Work out the finished part from the listing and answer in its coordinate system (mm). A direction names the side the tool comes from. Round coordinates to 2 decimals unless told otherwise and drop trailing zeros. Write each loop counter-clockwise with the first axis right and the second up, starting at its lowest first coordinate (ties: lowest second). Pieces come first, ordered by that corner, then holes.
1. Determine the mould class of faces 1 (the face through (-6.889, -8.376, 1.479)), 2 (the face through (15.021, -7.951, 28.248)), 3 (the face through (-2, -1, 3)), 4 (the face through (-10.907, 15.021, 28.248)) for opening direction Z: pulls with the +Z half, pulls with the -Z half, needs draft (parallel to the pull), parting line crosses it, or undercut.
2. Flat-ended cylindrical pins translate along their axes: pin 1 Ø9 at (y, z) = (4, 17) entering from -X; pin 2 Ø2 at (x, z) = (-5.5, 13) entering from -Y; pin 3 Ø5 at (x, y) = (-9.43, -9.43) entering from -Z. Find the tip coordinate at first contact, or state that the pin passes through.
3. Find section A-A (x = -9). Write down the section's boundary in (y, z), and give its area (3 significant figures).
4. Find section D-D (z = 6). Write down the section's boundary in (x, y).
5. Find section B-B (y = -7.5). Write down the section's boundary in (x, z), and give its area (3 significant figures).
6. Straight lines are drawn through the part: probe 1 along X at (y, z) = (-1, 15); probe 2 along Z at (x, y) = (-3, 5.5). For each, find the intervals that lie inside material, in ascending order.
7. A tool of negligible diameter and unlimited length cuts with its end or side. For faces 5 (the face through (0, 0, 0)), 6 (the face through (13.5, -2, 18)), from which of +Z, -Z, +X, -X, +Y, -Y can it reach the whole face along a straight path? Write none if from no direction.
8. Find section C-C (x = -3). Write down the section's boundary in (y, z).
```python
from build123d import *

# Parameters (mm, degrees)
F0_W     = 33
F0_H     = 33
F1_DEPTH = 3
F2_W     = 30
F2_H     = 3
F2_W_2   = 3
F2_H_2   = 30
F3_DEPTH = 30
F6_R     = 2.75
F7_DEPTH = 3
F4_R     = 2.75
F8_DEPTH = 3
F5_R     = 2.75
F9_DEPTH = 3


with BuildPart() as f1:
    # F0 (on Top) → F1 (new body)
    with BuildSketch(Plane.XY):
        Rectangle(F0_W, F0_H)
    extrude(amount=F1_DEPTH)

    # F2 (on face) → F3 (join)
    with BuildSketch(Plane.XY.offset(3)):
        with Locations((-1.5, 15)):
            Rectangle(F2_W, F2_H)
        with Locations((15, 15)):
            Rectangle(F2_W_2, F2_H)
        with Locations((15, -1.5)):
            Rectangle(F2_W_2, F2_H_2)
    extrude(amount=F3_DEPTH)

    # F6 (on face) → F7 (cut)
    with BuildSketch(Plane(origin=(0, 16.5, 0), x_dir=(-1, 0, 0), z_dir=(0, 1, 0))):
        with Locations((9.428932, 25.928932)):
            Circle(F6_R)
    extrude(amount=-F7_DEPTH, mode=Mode.SUBTRACT)

    # F4 (on face) → F8 (cut)
    with BuildSketch(Plane(origin=(0, 0, 0), x_dir=(1, 0, 0), z_dir=(0, 0, -1))):
        with Locations((-9.428932, 9.428932)):
            Circle(F4_R)
    extrude(amount=-F8_DEPTH, mode=Mode.SUBTRACT)

    # F5 (on face) → F9 (cut)
    with BuildSketch(Plane.YZ.offset(16.5)):
        with Locations((-9.428932, 25.928932)):
            Circle(F5_R)
    extrude(amount=-F9_DEPTH, mode=Mode.SUBTRACT)


solid = f1.part
```
Worked answers:
1. face 1: needs draft
1. face 2: undercut
1. face 3: pulls with the +Z half
1. face 4: undercut
2. pin 1: stops at x = 13.5
2. pin 2: stops at y = 13.5
2. pin 3: passes through
3. outline: (-16.5, 0) - (-12.15, 0) - (-12.15, 3) - (-16.5, 3) - close; (-6.71, 0) - (16.5, 0) - (16.5, 23.21) - (13.5, 23.21) - (13.5, 3) - (-6.71, 3) - close; (13.5, 28.65) - (16.5, 28.65) - (16.5, 33) - (13.5, 33) - close
3. area: 156 mm2
4. outline: (-16.5, 13.5) - (13.5, 13.5) - (13.5, -16.5) - (16.5, -16.5) - (16.5, 16.5) - (-16.5, 16.5) - close
5. outline: (-16.5, 0) - (-11.39, 0) - (-11.39, 3) - (-16.5, 3) - close; (-7.47, 0) - (16.5, 0) - (16.5, 23.97) - (13.5, 23.97) - (13.5, 3) - (-7.47, 3) - close; (13.5, 27.89) - (16.5, 27.89) - (16.5, 33) - (13.5, 33) - close
5. area: 165 mm2
6. probe 1: x = 13.5 to 16.5
6. probe 2: z = 0 to 3
7. face 5: -Z, +X, -X, +Y, -Y
7. face 6: +Z, -X, -Y
8. outline: (-16.5, 0) - (16.5, 0) - (16.5, 33) - (13.5, 33) - (13.5, 3) - (-16.5, 3) - close
